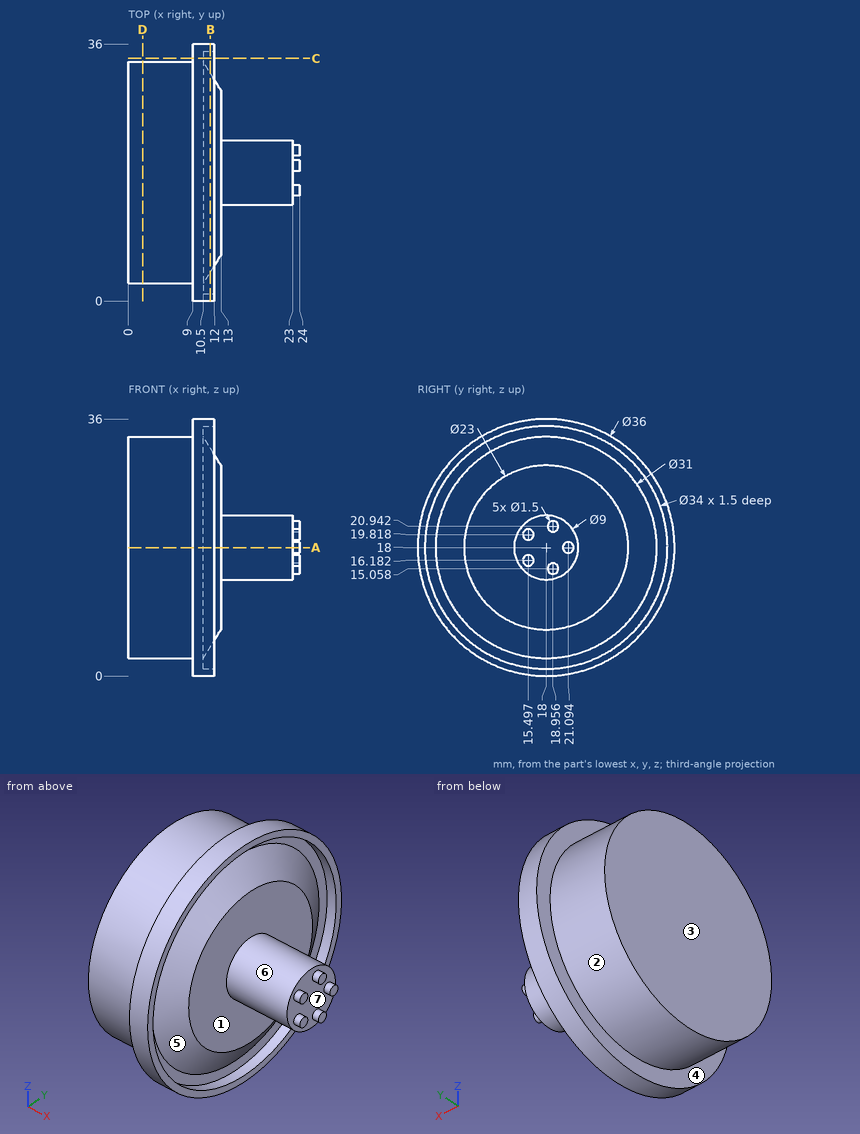
For this review, use the dimensioned drawing (mm, ordinates from the lowest corner) and the shaded views. A direction names the side the tool comes from. Coordinates: 2 decimals unless noted, no trailing zeros. Loops run counter-clockwise (first coordinate to the right, second up) from the corner with the lowest first, then second, coordinate; pieces in that order, holes last. Notation, with made-up numbers: (-3, 65) -> (37, 65) arc R7 cw to (37, 78) -> close; hole circle Ø2 at (83.25, 3.5). An arc over 180 degrees is marked (long way). Write each question's results on one line, items separated by ' | '.
Q1. Add section C-C, the plane y = 34. State the section outline as (x, z) points (1 decimal).
Taken from the geometry:
outline: (9, 9.8) -> (12, 9.8) -> (12, 12.3) -> (10.5, 12.3) -> (10.5, 23.7) -> (12, 23.7) -> (12, 26.2) -> (9, 26.2) -> close
Q2. Add section A-A, the plane z = 18. State the section outline as (x, y) points, then the cut area to 3 significant figures.
Taken from the geometry:
outline: (0, 2.5) -> (9, 2.5) -> (9, 0) -> (12, 0) -> (12, 1) -> (10.5, 1) -> (10.5, 2.5) -> (13, 6.5) -> (13, 13.5) -> (23, 13.5) -> (23, 20.34) -> (24, 20.34) -> (24, 21.84) -> (23, 21.84) -> (23, 22.5) -> (13, 22.5) -> (13, 29.5) -> (10.5, 33.5) -> (10.5, 35) -> (12, 35) -> (12, 36) -> (9, 36) -> (9, 33.5) -> (0, 33.5) -> close | area: 495 mm²
Q3. Mouldability with a two-part tool opening along Z and no side actions: class the marked faces 4, 5, 6 and 7 as +Z half, -Z half, draft (parallel to the pull), parting line (faces both ways), or undercut.
Taken from the geometry:
face 4: draft | face 5: undercut | face 6: parting line | face 7: undercut
Q4. Add section D-D, the plane x = 2. State the section outline as (y, z) points.
Taken from the geometry:
outline: circle Ø31 at (18, 18)
Q5. Add section B-B, the plane x = 11.5. State the section outline as (y, z) points, then the cut area to 3 significant figures.
Taken from the geometry:
outline: circle Ø36 at (18, 18); circle Ø27.8 at (18, 18); hole circle Ø34 at (18, 18) | area: 717 mm²
Q6. Machinability: for the marked faces 1, 2 and 3, which of the approach directions +Z, -Z, +X, -X, +Y, -Y give a long, thin tool a straight path to every point of the face, cutting with its end or side? Answer none if there is none.
Taken from the geometry:
face 1: +X | face 2: -X | face 3: +Z, -Z, -X, +Y, -Y
Q7. To check wall thickness, follow line 1 along Y through (x, z) = (10.95, 18); line 2 along Y through (x, z) = (11.35, 18); line 3 along X through (y, z) = (6.5, 29). State the ranges of each line that lie inside material, in increasing order. Write a range as [from, to].
Taken from the geometry:
line 1: [0, 1], [3.22, 32.78], [35, 36] | line 2: [0, 1], [3.86, 32.14], [35, 36] | line 3: [9, 10.5]
Q8. For pin 1 Ø6 at (x, y) = (18, 23) entering from +Z; pin 2 Ø4 at (x, z) = (9.5, 25) entering from -Y; pin 3 Ø12 at (x, z) = (13, 20.5) entering from -Y, all flat-tipped, find the tip position at first contact; note any pin that passes through.
Taken from the geometry:
pin 1: z = 22.03 | pin 2: y = 0.71 | pin 3: y = 0
